Work out the finished part from the listing and answer in its coordinate system (mm). Face numbers are marked on the shaded views. Coordinates: 2 decimals unless noted, no trailing zeros. Order: outer loops, then holes, each group sorted by start corner. A loop starts at its lowest first (then second) coordinate and runs counter-clockwise, first axis right, second up. Notation, with made-up numbers: M -36.75,-1.75 L -15.75,-1.75 A10 ccw -15.75,15.25 Z; hole C 67.5,37.5 d2. An arc over 180 degrees is marked long. Write item = value, one per line. Start each with the question number.
Q1. Determine the mould class of the marked faces 1, 2, 3 and 4 for opening direction Y: released by +Y, released by -Y, zero draft, split by the parting line, or undercut.
Q2. Straight lines are drawn through the part: line 1 along Y through (x, z) = (0, 0.75); line 2 along Y through (x, z) = (0.25, -2); line 3 along Z through (x, y) = (1.25, 25). For each, find the intervals that lie inside material, in ascending order.
Q3. Each of these flat-tipped pins is pushed along its axis until it touches: P1, Ø5, axis at x = -1, y = 45, coming from the -Z side; P2, Ø2.5, axis at x = 0, y = 49, coming from the +Z side. Where does it stop, or does it pass through?
Q4. Find section C-C on y = 11. Give the vertices of the cut face in (x, z).
Q5. Find section A-A on z = 1.5. Give the vertices of the cut face in (x, y), and give its area (3 significant figures).
Q6. Find section B-B on x = 0. Give the vertices of the cut face in (y, z), and give its area (3 significant figures).
Q7. Find section D-D on z = -1.25. Give the vertices of the cut face in (x, y), and give its area (3 significant figures).
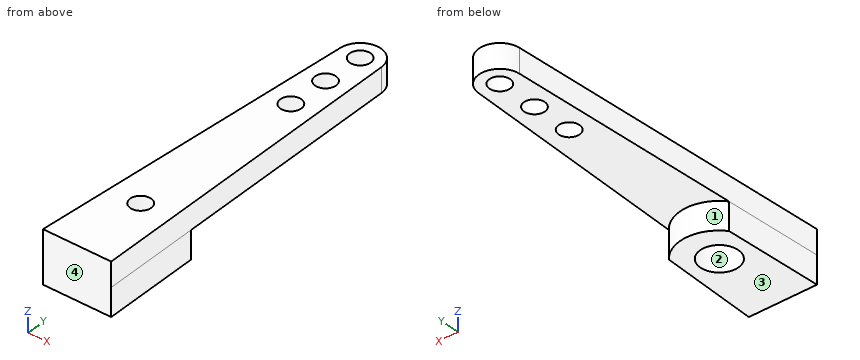
```python
from build123d import *

# Parameters (mm, degrees)
SKETCH_1_R          = 1.5
SKETCH_1_R_2        = 2.75
EXTRUDE_1_DEPTH     = 3.5
EXTRUDE_2_DEPTH     = 4
EXTRUDE_START       = -5
SKETCH_4_R          = 2.75
EXTRUDE_3_DEPTH     = 5
SKETCH_5_R          = 2.75
CUT_EXTRUDE_2_DEPTH = 4
SKETCH_6_R          = 1.5
CUT_EXTRUDE_3_DEPTH = 4


with BuildPart() as part:
    # 草图1 → 凸台-拉伸1 (new body)
    with BuildSketch(Plane.XY):
        with BuildLine():
            Line((-5, 0), (5, 0))
            Line((5, 0), (2.997510367, 49.122194935))
            ThreePointArc((2.997510367, 49.122194935), (0, 52), (-2.997510367, 49.122194935))
            Line((-2.997510367, 49.122194935), (-5, 0))
        make_face()
        with Locations((0, 49)):
            Circle(SKETCH_1_R, mode=Mode.SUBTRACT)
        with Locations((0, 43)):
            Circle(SKETCH_1_R, mode=Mode.SUBTRACT)
        with Locations((0, 37)):
            Circle(SKETCH_1_R, mode=Mode.SUBTRACT)
        with Locations((0, 11)):
            Circle(SKETCH_1_R_2, mode=Mode.SUBTRACT)
    extrude(amount=EXTRUDE_1_DEPTH)

    # 草图2 → 凸台-拉伸2 (add)
    with BuildSketch(Plane(origin=(0, 0, 0), x_dir=(-1, 0, 0), z_dir=(0, 0, -1))):
        with BuildLine():
            Line((5, 0), (4.407228658, 14.541013804))
            ThreePointArc((4.407228658, 14.541013804), (0, 16.653533692), (-4.407228658, 14.541013804))
            Line((-4.407228658, 14.541013804), (-5, 0))
            Line((-5, 0), (5, 0))
        make_face()
    extrude(amount=EXTRUDE_2_DEPTH)

    # 草图4 → 凸台-拉伸3 (add)
    with BuildSketch(Plane.XY.offset(3.5).offset(EXTRUDE_START)):
        with Locations((0, 11)):
            Circle(SKETCH_4_R)
    extrude(amount=EXTRUDE_3_DEPTH)

    # 草图5 → 切除-拉伸2 (cut)
    with BuildSketch(Plane(origin=(0, 0, -4), x_dir=(-1, 0, 0), z_dir=(0, 0, -1))):
        with Locations((0, 11)):
            Circle(SKETCH_5_R)
    extrude(amount=-CUT_EXTRUDE_2_DEPTH, mode=Mode.SUBTRACT)

    # 草图6 → 切除-拉伸3 (cut)
    with BuildSketch(Plane(origin=(0, 0, 0), x_dir=(-1, 0, 0), z_dir=(0, 0, -1))):
        with Locations((0, 11)):
            Circle(SKETCH_6_R)
    extrude(amount=-CUT_EXTRUDE_3_DEPTH, mode=Mode.SUBTRACT)


solid = part.part
```
Findings below:
q1.face_1 = released by +Y
q1.face_2 = undercut
q1.face_3 = zero draft
q1.face_4 = released by -Y
q2.line_1 = 0 to 9.5, 12.5 to 35.5, 38.5 to 41.5, 44.5 to 47.5, 50.5 to 52
q2.line_2 = 0 to 8.26, 13.74 to 16.65
q2.line_3 = 0 to 3.5
q3.P1 = 0
q3.P2 = through
q4.outline = M -4.55,-4 L -2.75,-4 L -2.75,0 L -1.5,0 L -1.5,3.5 L -4.55,3.5 Z; M 1.5,0 L 2.75,0 L 2.75,-4 L 4.55,-4 L 4.55,3.5 L 1.5,3.5 Z
q5.outline = M -5,0 L 5,0 L 3,49.12 A3 ccw -3,49.12 Z; hole C 0,11 d3; hole C 0,37 d3; hole C 0,43 d3; hole C 0,49 d3
q5.area = 378 mm^2
q6.outline = M 0,-4 L 8.25,-4 L 8.25,0 L 9.5,0 L 9.5,3.5 L 0,3.5 Z; M 12.5,0 L 13.75,0 L 13.75,-4 L 16.65,-4 L 16.65,0 L 35.5,0 L 35.5,3.5 L 12.5,3.5 Z; M 38.5,0 L 41.5,0 L 41.5,3.5 L 38.5,3.5 Z; M 44.5,0 L 47.5,0 L 47.5,3.5 L 44.5,3.5 Z; M 50.5,0 L 52,0 L 52,3.5 L 50.5,3.5 Z
q6.area = 185 mm^2
q7.outline = M -5,0 L 5,0 L 4.41,14.54 A5.65 ccw -4.41,14.54 Z; hole C 0,11 d5.5
q7.area = 126 mm^2
